Here's how the part is built. I have some questions about the finished solid (model axes, mm). A direction names the side the tool comes from. Give positions to 0.01 mm unless a question says otherwise; leave off trailing zeros. Loops run counter-clockwise (first coordinate to the right, second up) from the corner with the lowest first, then second, coordinate; pieces in that order, holes last. Notation, with made-up numbers: (-14, 39) -> (17, 39) arc R22 cw to (17, 55) -> close; hole circle Ø7 at (86, -20.5). An arc over 180 degrees is marked (long way). Answer in a Markdown table with one row per item. Add a question column.
Item 1: For P1, Ø8, axis at x = 28, y = 43.5, coming from the +Z side; P2, Ø5, axis at x = -6, y = -10, coming from the -Z side; P3, Ø1, axis at x = 47.5, y = 9, coming from the -Z side, each with a flat end and sliding along its axis, tell me the tip position at first contact or that it passes through.
Item 2: If I drill on line 1 (Y direction, x = 18, z = 23.5); line 2 (Z direction, x = 54, y = 28); line 3 (Y direction, x = 44, z = 30.5), over which ranges is the centre line in solid material (lowest first)?
Item 3: We'd pull the mould along Z, two halves only. Please class faces 1 (the face through (29.93, -79.845, -41.53)), 2 (the face through (30.42, 39.994, -0.687)), 3 (the face through (60, 1, 1)), 4 (the face through (30.42, -25.68, -6.51)): released by +Z, released by -Z, zero draft, split by the parting line, or undercut.
Item 4: Which directions (+Z, -Z, +X, -X, +Y, -Y) give clear straight access to the entire face, cutting with the end or side of a thin tool? Please do faces 5 (the face through (-32.06, -9.76, 2.17)), 6 (the face through (30.42, -19.4, 34.98)).
Item 5: If we section it at B-B (y = 0): Write out the boundary of the cut face in (x, z).
Item 6: If we section it at C-C (x = 45.5): Write out the boundary of the cut face in (y, z).
Item 7: If we section it at A-A (z = 0): Write out the boundary of the cut face in (x, y).
Item 8: If we section it at D-D (x = -10.5): Write out the boundary of the cut face in (y, z), then the cut area to 3 significant figures.
```python
from build123d import *
from build123d.topology import SkipClean

# Parameters (mm, degrees)
SKETCH1_R           = 90
BOSS_EXTRUDE1_DEPTH = 60
FILLET2_R           = 25
CUT_EXTRUDE5_DEPTH  = 141.712472859
SKETCH8_R           = 10
BOSS_EXTRUDE2_DEPTH = 124
SKETCH9_R           = 12.595659068
BOSS_EXTRUDE3_DEPTH = 61


with BuildPart() as part:
    # Sketch1 → Boss-Extrude1 (new body)
    with BuildSketch(Plane(origin=(0, 0, 0), x_dir=(0, 0, -1), z_dir=(1, 0, 0))):
        Circle(SKETCH1_R)
    extrude(amount=BOSS_EXTRUDE1_DEPTH)

    # Fillet2
    fillet2_edges = [part.edges().sort_by_distance(p)[0] for p in [
        (0, 0, 90),
        (60, 0, 90),
    ]]
    fillet(fillet2_edges, radius=FILLET2_R)

    # Sketch3 → Cut-Extrude5 (cut, through all)
    with BuildSketch(Plane(origin=(60, 0, 0), x_dir=(0, 0, -1), z_dir=(1, 0, 0))):
        with BuildLine():
            Line((-9.829866808, 38.773363519), (-2.457466702, 9.69334088))
            ThreePointArc((-2.457466702, 9.69334088), (0.135090676, 9.999087484), (2.718441847, 9.6234128))
            Line((2.718441847, 9.6234128), (10.873767388, 38.493651201))
            ThreePointArc((10.873767388, 38.493651201), (0.540362703, 39.996349935), (-9.829866808, 38.773363519))
        make_face()
        with BuildLine():
            Line((28.663784394, 27.89959613), (7.165946098, 6.974899033))
            ThreePointArc((7.165946098, 6.974899033), (8.727009114, 4.882551785), (9.69334088, 2.457466702))
            Line((9.69334088, 2.457466702), (38.773363519, 9.829866808))
            ThreePointArc((38.773363519, 9.829866808), (34.908036454, 19.53020714), (28.663784394, 27.89959613))
        make_face()
        with BuildLine():
            Line((38.493651201, -10.873767388), (9.6234128, -2.718441847))
            ThreePointArc((9.6234128, -2.718441847), (8.591918438, -5.116535699), (6.974899033, -7.165946098))
            Line((6.974899033, -7.165946098), (27.89959613, -28.663784394))
            ThreePointArc((27.89959613, -28.663784394), (34.367673751, -20.466142796), (38.493651201, -10.873767388))
        make_face()
        with BuildLine():
            ThreePointArc((2.457466702, -9.69334088), (-0.135090676, -9.999087484), (-2.718441847, -9.6234128))
            Line((-2.718441847, -9.6234128), (-10.873767388, -38.493651201))
            ThreePointArc((-10.873767388, -38.493651201), (-0.540362703, -39.996349935), (9.829866808, -38.773363519))
            Line((9.829866808, -38.773363519), (2.457466702, -9.69334088))
        make_face()
        with BuildLine():
            ThreePointArc((-7.165946098, -6.974899033), (-8.727009114, -4.882551785), (-9.69334088, -2.457466702))
            Line((-9.69334088, -2.457466702), (-38.773363519, -9.829866808))
            ThreePointArc((-38.773363519, -9.829866808), (-34.908036454, -19.53020714), (-28.663784394, -27.89959613))
            Line((-28.663784394, -27.89959613), (-7.165946098, -6.974899033))
        make_face()
        with BuildLine():
            ThreePointArc((-9.6234128, 2.718441847), (-8.591918438, 5.116535699), (-6.974899033, 7.165946098))
            Line((-6.974899033, 7.165946098), (-27.89959613, 28.663784394))
            ThreePointArc((-27.89959613, 28.663784394), (-34.367673751, 20.466142796), (-38.493651201, 10.873767388))
            Line((-38.493651201, 10.873767388), (-9.6234128, 2.718441847))
        make_face()
    extrude(amount=-CUT_EXTRUDE5_DEPTH, mode=Mode.SUBTRACT)

    # Sketch8 → Boss-Extrude2 (add)
    with SkipClean():  # the faces are left unmerged after this step: merging them gives an invalid solid
        with BuildSketch(Plane(origin=(60, 0, 0), x_dir=(0, 0, -1), z_dir=(1, 0, 0))):
            Circle(SKETCH8_R)
        extrude(amount=-BOSS_EXTRUDE2_DEPTH)

    # Sketch9 → Boss-Extrude3 (add)
    with BuildSketch(Plane(origin=(60, 0, 0), x_dir=(0, 0, -1), z_dir=(1, 0, 0))):
        Circle(SKETCH9_R)
    extrude(amount=-BOSS_EXTRUDE3_DEPTH)


solid = part.part
```
Recorded:
| question | item | result |
|---|---|---|
| 1 | P1 | stops at z = 80.87 |
| 1 | P2 | stops at z = -6.61 |
| 1 | P3 | stops at z = -86.47 |
| 2 | line 1 | y = -85.84 to -22.87, -5.96 to 6.64, 24.14 to 85.84 |
| 2 | line 2 | z = -76.27 to -7.91, 7.1 to 27.25, 28.57 to 76.27 |
| 2 | line 3 | y = -82.89 to -25.88, -7.73 to 8.62, 25.88 to 82.89 |
| 3 | face 1 | split by the parting line |
| 3 | face 2 | undercut |
| 3 | face 3 | zero draft |
| 3 | face 4 | undercut |
| 4 | face 5 | -X |
| 4 | face 6 | +X, -X |
| 5 | outline | (-64, -10) -> (-1, -10) -> (-1, -12.6) -> (0, -12.6) -> (0, -65) arc R25 ccw to (25, -90) -> (35, -90) arc R25 ccw to (60, -65) -> (60, 65) arc R25 ccw to (35, 90) -> (25, 90) arc R25 ccw to (0, 65) -> (0, 12.6) -> (-1, 12.6) -> (-1, 10) -> (-64, 10) -> close |
| 6 | outline | circle Ø175.38 at (0, 0); hole (-38.77, -9.83) -> (-12.21, -3.1) arc R12.6 cw to (-12.12, 3.42) -> (-38.49, 10.87) arc R40 ccw to start; hole (-28.66, -27.9) arc R40 ccw to (-10.87, -38.49) -> (-3.42, -12.12) arc R12.6 cw to (-9.03, -8.79) -> close; hole (-27.9, 28.66) -> (-8.79, 9.03) arc R12.6 cw to (-3.1, 12.21) -> (-9.83, 38.77) arc R40 ccw to start; hole (3.1, -12.21) -> (9.83, -38.77) arc R40 ccw to (27.9, -28.66) -> (8.79, -9.03) arc R12.6 cw to start; hole (3.42, 12.12) arc R12.6 cw to (9.03, 8.79) -> (28.66, 27.9) arc R40 ccw to (10.87, 38.49) -> close; hole (12.12, -3.42) -> (38.49, -10.87) arc R40 ccw to (38.77, 9.83) -> (12.21, 3.1) arc R12.6 cw to start |
| 7 | outline | (-64, -10) -> (-1, -10) -> (-1, -12.6) -> (60, -12.6) -> (60, 12.6) -> (-1, 12.6) -> (-1, 10) -> (-64, 10) -> close; (0, -65) arc R25 ccw to (25, -90) -> (35, -90) arc R25 ccw to (60, -65) -> (60, -40) -> (0, -40) -> close; (0, 40) -> (60, 40) -> (60, 65) arc R25 ccw to (35, 90) -> (25, 90) arc R25 ccw to (0, 65) -> close |
| 8 | outline | circle Ø20 at (0, 0) |
| 8 | area | 314 mm^2 |
